Read the model definition and answer for the solid it produces. Units are mm, in the model's axes. Face numbers are marked on the shaded views. A direction names the side the tool comes from. Give positions to 0.01 mm unless a question says otherwise; leave off trailing zeros. Write each loop counter-clockwise with the first axis right and the second up, starting at its lowest first coordinate (ties: lowest second). Pieces come first, ordered by that corner, then holes. Notation, with made-up numbers: (-39.75, -8.75) - (-2.75, -8.75) arc R38 ccw to (-2.75, 30.25) - close; hole circle Ø1 at (-22.5, 26). An arc over 180 degrees is marked (long way). Answer as CSV lines item,"result".
```python
from build123d import *

# Parameters (mm, degrees)
SKETCH1_W                               = 96.210678118
SKETCH1_H                               = 96.210678118
SKETCH1_R                               = 11
SKETCH1_R_2                             = 2
SKETCH1_R_3                             = 4.25
MAIN_BODY_DEPTH                         = 60
MAIN_MILL_CUT_DEPTH                     = 48
SKETCH2_R                               = 3.625
MOTOR_MOUNT_BOLT_HEAD_COUNTERSINK_DEPTH = 54


with BuildPart() as part:
    # Sketch1 → main body (new body)
    with BuildSketch(Plane(origin=(0, 0, 0), x_dir=(1, 0, 0), z_dir=(0, 1, 0))):
        Rectangle(SKETCH1_W, SKETCH1_H)
        with Locations(Location((0, 0, 0), (0, 0, 270))):
            Circle(SKETCH1_R, mode=Mode.SUBTRACT)
        with Locations(Location((0, 15, 0), (0, 0, 270))):
            Circle(SKETCH1_R_2, mode=Mode.SUBTRACT)
        with Locations(Location((35.355339059, 35.355339059, 0), (0, 0, 270))):
            Circle(SKETCH1_R_3, mode=Mode.SUBTRACT)
        with Locations(Location((12.990381057, 7.5, 0), (0, 0, 270))):
            Circle(SKETCH1_R_2, mode=Mode.SUBTRACT)
        with Locations(Location((12.990381057, -7.5, 0), (0, 0, 270))):
            Circle(SKETCH1_R_2, mode=Mode.SUBTRACT)
        with Locations(Location((0, -15, 0), (0, 0, 270))):
            Circle(SKETCH1_R_2, mode=Mode.SUBTRACT)
        with Locations(Location((-12.990381057, -7.5, 0), (0, 0, 270))):
            Circle(SKETCH1_R_2, mode=Mode.SUBTRACT)
        with Locations(Location((-12.990381057, 7.5, 0), (0, 0, 270))):
            Circle(SKETCH1_R_2, mode=Mode.SUBTRACT)
        with Locations(Location((35.355339059, -35.355339059, 0), (0, 0, 270))):
            Circle(SKETCH1_R_3, mode=Mode.SUBTRACT)
        with Locations(Location((-35.355339059, -35.355339059, 0), (0, 0, 270))):
            Circle(SKETCH1_R_3, mode=Mode.SUBTRACT)
        with Locations(Location((-35.355339059, 35.355339059, 0), (0, 0, 270))):
            Circle(SKETCH1_R_3, mode=Mode.SUBTRACT)
    extrude(amount=MAIN_BODY_DEPTH)

    # Sketch4 → main mill cut (cut)
    with BuildSketch(Plane(origin=(0, 60, 0), x_dir=(1, 0, 0), z_dir=(0, 1, 0))):
        Polygon((-22.605339059, 48.105339059), (22.605339059, 48.105339059), (22.605339059, 22.605339059), (48.105339059, 22.605339059), (48.105339059, -22.605339059), (22.605339059, -22.605339059), (22.605339059, -48.105339059), (-22.605339059, -48.105339059), (-22.605339059, -22.605339059), (-48.105339059, -22.605339059), (-48.105339059, 22.605339059), (-22.605339059, 22.605339059), align=None)
    extrude(amount=-MAIN_MILL_CUT_DEPTH, mode=Mode.SUBTRACT)

    # Sketch2 → motor mount bolt head countersink (cut)
    with BuildSketch(Plane(origin=(0, 60, 0), x_dir=(1, 0, 0), z_dir=(0, 1, 0))):
        with Locations(Location((12.990381057, 7.5, 0), (0, 0, 270))):
            Circle(SKETCH2_R)
        with Locations(Location((0, 15, 0), (0, 0, 270))):
            Circle(SKETCH2_R)
        with Locations(Location((12.990381057, -7.5, 0), (0, 0, 270))):
            Circle(SKETCH2_R)
        with Locations(Location((0, -15, 0), (0, 0, 270))):
            Circle(SKETCH2_R)
        with Locations(Location((-12.990381057, -7.5, 0), (0, 0, 270))):
            Circle(SKETCH2_R)
        with Locations(Location((-12.990381057, 7.5, 0), (0, 0, 270))):
            Circle(SKETCH2_R)
    extrude(amount=-MOTOR_MOUNT_BOLT_HEAD_COUNTERSINK_DEPTH, mode=Mode.SUBTRACT)


solid = part.part
```
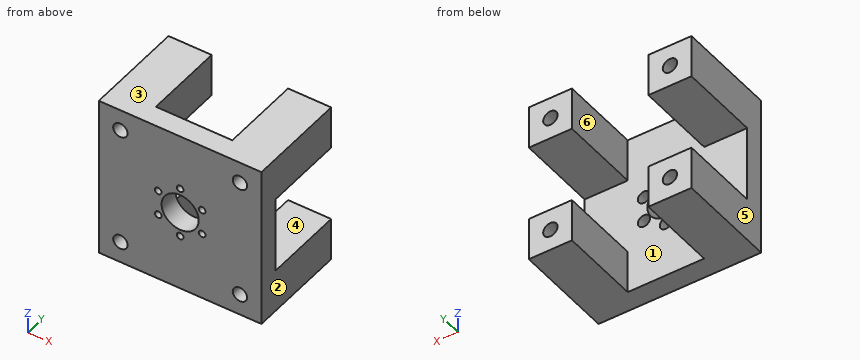
(1) The mould has two halves that part along X. Classify the marked faces 1, 2 and 3: +X half, -X half, draft (parallel to the pull), parting line (faces both ways), or undercut.
Worked out:
face 1,"undercut"
face 2,"+X half"
face 3,"draft"
(2) A cutting plane is placed at B-B (x = 0). Write down the section's boundary in (y, z) (3 decimals).
Worked out:
outline,"(0, -48.105) - (12, -48.105) - (12, -18.625) - (6, -18.625) - (6, -17) - (0, -17) - close; (0, -13) - (6, -13) - (6, -11.375) - (12, -11.375) - (12, -11) - (0, -11) - close; (0, 11) - (12, 11) - (12, 11.375) - (6, 11.375) - (6, 13) - (0, 13) - close; (0, 17) - (6, 17) - (6, 18.625) - (12, 18.625) - (12, 48.105) - (0, 48.105) - close"
(3) A cutting plane is placed at A-A (z = 0). Write down the section's boundary in (x, y).
Worked out:
outline,"(-48.11, 0) - (-11, 0) - (-11, 12) - (-48.11, 12) - close; (11, 0) - (48.11, 0) - (48.11, 12) - (11, 12) - close"
(4) A cutting plane is placed at D-D (x = 28). Write down the section's boundary in (y, z), and give its area (3 significant figures).
Worked out:
outline,"(0, -48.11) - (60, -48.11) - (60, -22.61) - (12, -22.61) - (12, 22.61) - (60, 22.61) - (60, 48.11) - (0, 48.11) - close"
area,"3,600 mm^2"
(5) Each of these flat-tipped pins is pushed along its axis until it touches: P1, Ø6, axis at x = 0, z = 15, coming from the +Y side; P2, Ø7, axis at x = -35.36, z = 35.36, coming from the +Y side; P3, Ø8.5, axis at x = 12.99, z = 7.5, coming from the +Y side. Where does it stop, or does it pass through?
Worked out:
P1,"stops at y = 6"
P2,"passes through"
P3,"stops at y = 12"
(6) Find the intervals of material crossed by L1, parallel to Z at x = 35.5, y = 41; L2, parallel to X at y = 3.9, z = -7.5; L3, parallel to X at y = 24, z = -31.5, in increasing order.
Worked out:
L1,"z = -48.11 to -39.6, -31.11 to -22.61, 22.61 to 31.11, 39.6 to 48.11"
L2,"x = -48.11 to -14.99, -10.99 to -8.05, 8.05 to 10.99, 14.99 to 48.11"
L3,"x = -48.11 to -37.14, -33.57 to -22.61, 22.61 to 33.57, 37.14 to 48.11"
(7) For the marked faces 4, 5 and 6, determine the directions among +Z, -Z, +X, -X, +Y, -Y from which every point of the face is accessible in a straight line to the end or side of a thin tool.
Worked out:
face 4,"+X, -X, +Y"
face 5,"+Z, -Z, -X, +Y, -Y"
face 6,"+Z, -Z, +Y"
(8) A cutting plane is placed at C-C (y = 33.5). Write down the section's boundary in (x, z), and give its area (3 significant figures).
Worked out:
outline,"(-48.11, -48.11) - (-22.61, -48.11) - (-22.61, -22.61) - (-48.11, -22.61) - close; (-48.11, 22.61) - (-22.61, 22.61) - (-22.61, 48.11) - (-48.11, 48.11) - close; (22.61, -48.11) - (48.11, -48.11) - (48.11, -22.61) - (22.61, -22.61) - close; (22.61, 22.61) - (48.11, 22.61) - (48.11, 48.11) - (22.61, 48.11) - close; hole circle Ø8.5 at (-35.36, -35.36); hole circle Ø8.5 at (-35.36, 35.36); hole circle Ø8.5 at (35.36, -35.36); hole circle Ø8.5 at (35.36, 35.36)"
area,"2,370 mm^2"
